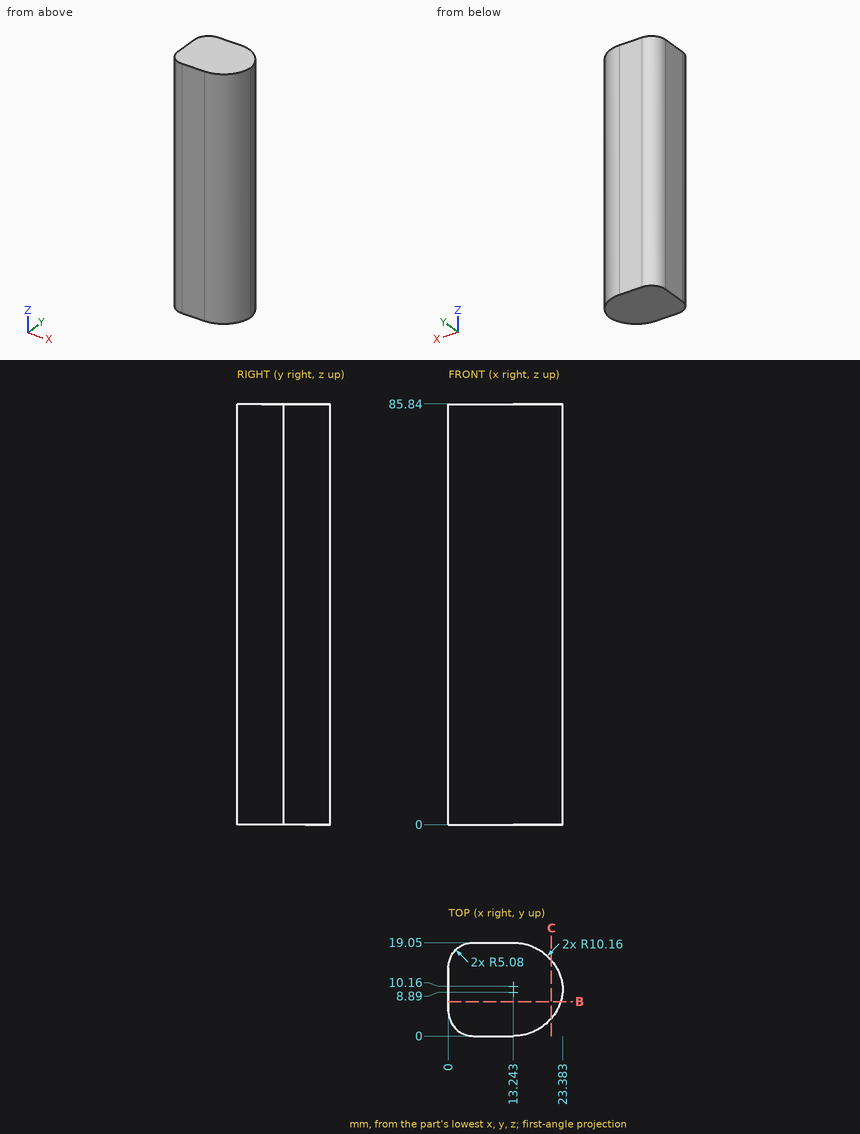
Check sheet for the drawn part. Datum: minimum x, y, z corner. Units: mm. Round coordinates to 2 decimals unless told otherwise and drop trailing zeros. Loops run counter-clockwise (first coordinate to the right, second up) from the corner with the lowest first, then second, coordinate; pieces in that order, holes last.
Item 1: Cross-section at B-B on y = 7. Record the boundary of the cut face in (x, z).
Item 2: Thickness scan on line 1 (Y direction, x = 13.5, z = 65); line 2 (X direction, y = 9, z = 54.5) (1 decimal); line 3 (Y direction, x = 17.5, z = 5) (1 decimal). Record the ranges inside material, lowest first.
Item 3: Gauge pin test, flat ends, axial feed: pin 1 (4 mm diameter, centred on y = 15.5, z = 52, fed in from +X); pin 2 (6 mm diameter, centred on y = 5.5, z = 21.5, fed in from +X); pin 3 (4 mm diameter, centred on y = 17, z = 9.5, fed in from -X) (1 decimal). Record the tip position at first contact, or that the pin passes through.
Item 4: Cross-section at C-C on x = 21. Record the boundary of the cut face in (y, z), then the cut area to 3 significant figures.
Answer sheet:
1. outline: (0, 0) - (22.9, 0) - (22.9, 85.84) - (0, 85.84) - close
2. line 1: y = 0 to 19.05
2. line 2: x = 0 to 23.3
2. line 3: y = 0.9 to 18.1
3. pin 1: stops at x = 22.3
3. pin 2: stops at x = 23.27
3. pin 3: stops at x = 0.1
4. outline: (3.6, 0) - (15.45, 0) - (15.45, 85.84) - (3.6, 85.84) - close
4. area: 1,020 mm2
